```python
from build123d import *

# Parameters (mm, degrees)
SKETCH_1_W          = 125
SKETCH_1_H          = 70
EXTRUDE_1_DEPTH     = 5
SKETCH_2_W          = 7.5
SKETCH_2_H          = 5
CUT_EXTRUDE_1_DEPTH = 70
EXTRUDE_START       = -70
EXTRUDE_2_DEPTH     = 70
CUT_EXTRUDE_2_REACH = 145.713
SKETCH_5_R          = 11.2
EXTRUDE_3_DEPTH     = 20
SKETCH_7_R          = 1.5
CUT_EXTRUDE_3_DEPTH = 10
CUT_EXTRUDE_4_REACH = 146.193
SKETCH_8_R          = 1.5
SKETCH_9_R          = 3
SKETCH_9_R_2        = 1.5
CUT_EXTRUDE_5_DEPTH = 3.5
SKETCH_11_R         = 1.5
CUT_EXTRUDE_6_DEPTH = 10
CUT_EXTRUDE_7_REACH = 146.193
SKETCH_12_R         = 1
FILLET_1_R          = 4
SKETCH_14_R         = 1.5
CUT_EXTRUDE_8_DEPTH = 10


# Read off the part's stored shape, not the designer's step: 凸台-拉伸2
with BuildPart() as part:
    # 草图1 → 凸台-拉伸1 (new body)
    with BuildSketch(Plane(origin=(0, 0, 0), x_dir=(1, 0, 0), z_dir=(0, 1, 0))):
        with Locations((62.5, 35)):
            Rectangle(SKETCH_1_W, SKETCH_1_H)
    extrude(amount=EXTRUDE_1_DEPTH)

    # 草图2 → 切除-拉伸1 (cut)
    with BuildSketch(Plane.XY):
        with Locations((3.75, 2.5)):
            Rectangle(SKETCH_2_W, SKETCH_2_H)
    extrude(amount=-CUT_EXTRUDE_1_DEPTH, mode=Mode.SUBTRACT)

    # 凸台-拉伸2 outline → 凸台-拉伸2 (add)
    with BuildSketch(Plane.XY.offset(EXTRUDE_START)):
        with BuildLine():
            Line((125, -5), (125, 0))
            Line((125, 0), (7.5, 0))
            Line((7.5, 0), (7.500013395, -11.329987981))
            Line((7.500013395, -11.329987981), (8.200014526, -11.329987981))
            ThreePointArc((8.200014526, -11.329987981), (18.500017961, -4.191325734), (28.800021395, -11.329987981))
            Line((28.800021395, -11.329987981), (30.200014526, -11.329987981))
            ThreePointArc((30.200014526, -11.329987981), (40.500017961, -4.191325734), (50.800021395, -11.329987981))
            Line((50.800021395, -11.329987981), (52.200014526, -11.329987981))
            ThreePointArc((52.200014526, -11.329987981), (62.500017961, -4.191325734), (72.800021395, -11.329987981))
            Line((72.800021395, -11.329987981), (74.200014526, -11.329987981))
            ThreePointArc((74.200014526, -11.329987981), (84.500017961, -4.191325734), (94.800021395, -11.329987981))
            Line((94.800021395, -11.329987981), (96.200014526, -11.329987981))
            ThreePointArc((96.200014526, -11.329987981), (102.083615638, -5.116833662), (110.639689418, -5))
            Line((110.639689418, -5), (125, -5))
        make_face()
    extrude(amount=EXTRUDE_2_DEPTH)

    # 草图5 → 切除-拉伸2 (cut, up to next)
    with BuildSketch(Plane.XY, mode=Mode.PRIVATE) as cut_extrude_2_sk1:
        with Locations((18.500017961, -15.191325734)):
            Circle(SKETCH_5_R)
    cut_extrude_2_tool1 = extrude(cut_extrude_2_sk1.sketch, amount=-CUT_EXTRUDE_2_REACH, mode=Mode.PRIVATE) & part.part
    # 草图5 → 切除-拉伸2 (cut, up to next)
    with BuildSketch(Plane.XY, mode=Mode.PRIVATE) as cut_extrude_2_sk2:
        with Locations((40.500017961, -15.191325734)):
            Circle(SKETCH_5_R)
    cut_extrude_2_tool2 = extrude(cut_extrude_2_sk2.sketch, amount=-CUT_EXTRUDE_2_REACH, mode=Mode.PRIVATE) & part.part
    # 草图5 → 切除-拉伸2 (cut, up to next)
    with BuildSketch(Plane.XY, mode=Mode.PRIVATE) as cut_extrude_2_sk3:
        with Locations((62.500017961, -15.191325734)):
            Circle(SKETCH_5_R)
    cut_extrude_2_tool3 = extrude(cut_extrude_2_sk3.sketch, amount=-CUT_EXTRUDE_2_REACH, mode=Mode.PRIVATE) & part.part
    # 草图5 → 切除-拉伸2 (cut, up to next)
    with BuildSketch(Plane.XY, mode=Mode.PRIVATE) as cut_extrude_2_sk4:
        with Locations((84.500017961, -15.191325734)):
            Circle(SKETCH_5_R)
    cut_extrude_2_tool4 = extrude(cut_extrude_2_sk4.sketch, amount=-CUT_EXTRUDE_2_REACH, mode=Mode.PRIVATE) & part.part
    # 草图5 → 切除-拉伸2 (cut, up to next)
    with BuildSketch(Plane.XY, mode=Mode.PRIVATE) as cut_extrude_2_sk5:
        with Locations((106.500017961, -15.191325734)):
            Circle(SKETCH_5_R)
    cut_extrude_2_tool5 = extrude(cut_extrude_2_sk5.sketch, amount=-CUT_EXTRUDE_2_REACH, mode=Mode.PRIVATE) & part.part
    add(cut_extrude_2_tool1.solids().sort_by_distance((18.500018, -15.191326, 0))[0], mode=Mode.SUBTRACT)
    add(cut_extrude_2_tool2.solids().sort_by_distance((40.500018, -15.191326, 0))[0], mode=Mode.SUBTRACT)
    add(cut_extrude_2_tool3.solids().sort_by_distance((62.500018, -15.191326, 0))[0], mode=Mode.SUBTRACT)
    add(cut_extrude_2_tool4.solids().sort_by_distance((84.500018, -15.191326, 0))[0], mode=Mode.SUBTRACT)
    add(cut_extrude_2_tool5.solids().sort_by_distance((106.500018, -15.191326, 0))[0], mode=Mode.SUBTRACT)

    # 草图6 → 凸台-拉伸3 (add)
    with BuildSketch(Plane.XY):
        Polygon((7.5, 5), (125, 5), (125, -3.991325734), (125, -5), (117.700017961, -5), (117.700017961, -3.991325734), (7.5, -3.991325734), align=None)
    extrude(amount=EXTRUDE_3_DEPTH)

    # 草图7 → 切除-拉伸3 (cut)
    with BuildSketch(Plane(origin=(0, 0, -70), x_dir=(-1, 0, 0), z_dir=(0, 0, -1))):
        with Locations((-29.49999102, -1)):
            Circle(SKETCH_7_R)
        with Locations((-95.50000898, -1)):
            Circle(SKETCH_7_R)
    extrude(amount=-CUT_EXTRUDE_3_DEPTH, mode=Mode.SUBTRACT)

    # 草图8 → 切除-拉伸4 (cut, up to next)
    with BuildSketch(Plane(origin=(0, 5, 0), x_dir=(1, 0, 0), z_dir=(0, 1, 0)), mode=Mode.PRIVATE) as cut_extrude_4_sk1:
        with Locations(Location((121.35000898, 58, 0), (0, 0, 270))):
            Circle(SKETCH_8_R)
    cut_extrude_4_tool1 = extrude(cut_extrude_4_sk1.sketch, amount=-CUT_EXTRUDE_4_REACH, mode=Mode.PRIVATE) & part.part
    # 草图8 → 切除-拉伸4 (cut, up to next)
    with BuildSketch(Plane(origin=(0, 5, 0), x_dir=(1, 0, 0), z_dir=(0, 1, 0)), mode=Mode.PRIVATE) as cut_extrude_4_sk2:
        with Locations(Location((121.35000898, -8, 0), (0, 0, 270))):
            Circle(SKETCH_8_R)
    cut_extrude_4_tool2 = extrude(cut_extrude_4_sk2.sketch, amount=-CUT_EXTRUDE_4_REACH, mode=Mode.PRIVATE) & part.part
    add(cut_extrude_4_tool1.solids().sort_by_distance((121.350009, 5, -58))[0], mode=Mode.SUBTRACT)
    add(cut_extrude_4_tool2.solids().sort_by_distance((121.350009, 5, 8))[0], mode=Mode.SUBTRACT)

    # 草图9 → 切除-拉伸5 (cut)
    # profile 1 of 2: a face of its own
    with BuildSketch(Plane(origin=(0, 5, 0), x_dir=(1, 0, 0), z_dir=(0, 1, 0))):
        with Locations(Location((121.35000898, 58, 0), (0, 0, 270))):
            Circle(SKETCH_9_R)
        with Locations(Location((121.35000898, 58, 0), (0, 0, 270))):
            Circle(SKETCH_9_R_2, mode=Mode.SUBTRACT)
    # profile 2 of 2: a face of its own
    with BuildSketch(Plane(origin=(0, 5, 0), x_dir=(1, 0, 0), z_dir=(0, 1, 0))):
        with Locations(Location((121.35000898, -8, 0), (0, 0, 270))):
            Circle(SKETCH_9_R)
        with Locations(Location((121.35000898, -8, 0), (0, 0, 270))):
            Circle(SKETCH_9_R_2, mode=Mode.SUBTRACT)
    extrude(amount=-CUT_EXTRUDE_5_DEPTH, mode=Mode.SUBTRACT)

    # 草图11 → 切除-拉伸6 (cut)
    with BuildSketch(Plane.ZY.offset(-7.5)):
        with Locations((8, 0.504337133)):
            Circle(SKETCH_11_R)
        with Locations((-58, 0.504337133)):
            Circle(SKETCH_11_R)
    extrude(amount=-CUT_EXTRUDE_6_DEPTH, mode=Mode.SUBTRACT)

    # 草图12 → 切除-拉伸7 (cut, up to next)
    with BuildSketch(Plane(origin=(0, 5, 0), x_dir=(1, 0, 0), z_dir=(0, 1, 0)), mode=Mode.PRIVATE) as cut_extrude_7_sk1:
        with Locations(Location((110.558, 7.891, 0), (0, 0, 270))):
            Circle(SKETCH_12_R)
    cut_extrude_7_tool1 = extrude(cut_extrude_7_sk1.sketch, amount=-CUT_EXTRUDE_7_REACH, mode=Mode.PRIVATE) & part.part
    # 草图12 → 切除-拉伸7 (cut, up to next)
    with BuildSketch(Plane(origin=(0, 5, 0), x_dir=(1, 0, 0), z_dir=(0, 1, 0)), mode=Mode.PRIVATE) as cut_extrude_7_sk2:
        with Locations(Location((14.434, 7.891, 0), (0, 0, 270))):
            Circle(SKETCH_12_R)
    cut_extrude_7_tool2 = extrude(cut_extrude_7_sk2.sketch, amount=-CUT_EXTRUDE_7_REACH, mode=Mode.PRIVATE) & part.part
    add(cut_extrude_7_tool1.solids().sort_by_distance((110.558, 5, -7.891))[0], mode=Mode.SUBTRACT)
    add(cut_extrude_7_tool2.solids().sort_by_distance((14.434, 5, -7.891))[0], mode=Mode.SUBTRACT)

    # 圆角1
    # the kernel refuses this fillet: 4 mm, written as the material it takes off along each edge
    with BuildSketch(Plane(origin=(125, 5, -80), x_dir=(0, -1, 0), z_dir=(0, 0, 1))) as fillet_1_piece_1:
        with BuildLine():
            CenterArc((FILLET_1_R, -FILLET_1_R), FILLET_1_R, 90, 90)
            Line((0, -FILLET_1_R), (0, 0))
            Line((0, 0), (FILLET_1_R, 0))
        make_face()
    extrude(amount=110, mode=Mode.SUBTRACT)

    # 草图14 → 切除-拉伸8 (cut)
    with BuildSketch(Plane.XY.offset(20)):
        with Locations((62.5, 0.504337133)):
            Circle(SKETCH_14_R)
    extrude(amount=-CUT_EXTRUDE_8_DEPTH, mode=Mode.SUBTRACT)


solid = part.part
```
Can you work these out from the model? Positions are in its coordinate system, mm. A direction names the side the tool comes from. Give positions to 0.01 mm unless a question says otherwise; leave off trailing zeros. Order: outer loops, then holes, each group sorted by start corner. A loop starts at its lowest first (then second) coordinate and runs counter-clockwise, first axis right, second up. Notation, with made-up numbers: M -9.5,0.5 L 29.5,0.5 A15 cw 29.5,23.5 Z; hole C 77,-5 d5. An arc over 180 degrees is marked long. Write item = value, one per line. Start each with the question number.
Q1. Suppose I cut it at A-A (z = -58). Write out the boundary of the cut face in (x, y).
Q2. Will these pins go through, and if not, where does the flat tip stop? pin 1 Ø0.9 at (x, y) = (29.5, -1.5) entering from -Z; pin 2 Ø3 at (x, z) = (14.434, -7.891) entering from -Y; pin 3 Ø1.5 at (y, z) = (1, 8.5) entering from -X.
Q3. Suppose I cut it at B-B (y = -7.75). Write out the boundary of the cut face in (x, z).
Q4. Suppose I cut it at D-D (x = 22.5). Write out the boundary of the cut face in (y, z), plus the area to 3 significant figures.
Q5. I need wall thicknesses on probe 1 along Y at (x, z) = (62.5, 13); probe 2 along X at (y, z) = (-9.75, -5.5); probe 3 along X at (y, z) = (-6.5, -54). Which ranges of each line are inside material? Lowest first, please. Write a range as [from, to].
Q6. For faces 5 (the flat face through (10, -6, 0)), 6 (the cylindrical face through (12.43, -0.41, 6.81)), 7 (the flat face through (123, 1.5, 9)), 8 (the cylindrical face through (94, -1, -65)), which set-ups out of +Z, -Z, +X, -X, +Y, -Y let a thin tool reach every point of the face, with its end or its side?
Q7. Suppose I cut it at C-C (z = -34). Write out the boundary of the cut face in (x, y), plus the area to 3 significant figures.
Q8. We'd pull the mould along Y, two halves only. Please class faces 1 (the cylindrical face through (28, -1, -65)), 2 (the flat face through (30, -1, -60)), 3 (the flat face through (123, 1.5, -57)), 4 (the flat face through (67, 0, 20)): pulls with the +Y half, pulls with the -Y half, needs draft (parallel to the pull), parting line crosses it, or undercut.
Check result:
q1.outline = M 7.5,-11.33 L 7.99,-11.33 A11.2 cw 29.01,-11.33 L 29.99,-11.33 A11.2 cw 51.01,-11.33 L 51.99,-11.33 A11.2 cw 73.01,-11.33 L 73.99,-11.33 A11.2 cw 95.01,-11.33 L 95.99,-11.33 A11.2 cw 111.15,-5 L 119.85,-5 L 119.85,1.5 L 118.35,1.5 L 118.35,5 L 7.5,5 L 7.5,2 L 17.5,2 L 17.5,-1 L 7.5,-1 Z; M 122.85,-5 L 125,-5 L 125,1 A4 ccw 124.35,3.19 L 124.35,1.5 L 122.85,1.5 Z
q2.pin_1 = -60
q2.pin_2 = -5.47
q2.pin_3 = 17.5
q3.outline = M 7.5,-70 L 10.13,-70 L 10.13,0 L 7.5,0 Z; M 26.87,-70 L 32.13,-70 L 32.13,0 L 26.87,0 Z; M 48.87,-70 L 54.13,-70 L 54.13,0 L 48.87,0 Z; M 70.87,-70 L 76.13,-70 L 76.13,0 L 70.87,0 Z; M 92.87,-70 L 98.13,-70 L 98.13,0 L 92.87,0 Z
q4.outline = M -4.73,-70 L 5,-70 L 5,20 L -3.99,20 L -3.99,0 L -4.73,0 Z
q4.area = 861 mm2
q5.probe_1 = [-3.99, -1], [2, 5]
q5.probe_2 = [7.5, 8.71], [28.29, 30.71], [50.29, 52.71], [72.29, 74.71], [94.29, 96.71]
q5.probe_3 = [7.5, 11.44], [25.56, 33.44], [47.56, 55.44], [69.56, 77.44], [91.56, 99.44]
q6.face_5 = +Z, -X, -Y
q6.face_6 = -X
q6.face_7 = +Y
q6.face_8 = -Z
q7.outline = M 7.5,-11.33 L 7.99,-11.33 A11.2 cw 29.01,-11.33 L 29.99,-11.33 A11.2 cw 51.01,-11.33 L 51.99,-11.33 A11.2 cw 73.01,-11.33 L 73.99,-11.33 A11.2 cw 95.01,-11.33 L 95.99,-11.33 A11.2 cw 111.15,-5 L 125,-5 L 125,1 A4 ccw 121,5 L 7.5,5 L 7.5,0 Z
q7.area = 1,290 mm2
q8.face_1 = undercut
q8.face_2 = undercut
q8.face_3 = pulls with the +Y half
q8.face_4 = needs draft
